Work out the finished part from the listing and answer in its coordinate system (mm). A direction names the side the tool comes from. Coordinates: 2 decimals unless noted, no trailing zeros. Order: outer loops, then holes, each group sorted by start corner. A loop starts at its lowest first (then second) coordinate and runs counter-clockwise, first axis right, second up. Notation, with made-up numbers: M -15,-16.5 L 38,-16.5 A28 cw 38,21.5 Z; hole C 60,86 d9. An arc over 180 degrees is marked long. Use a Markdown table: item, result.
from build123d import *

# Parameters (mm, degrees)
F0_W      = 127
F0_H      = 127
F1_DEPTH  = 63.5
F1_FACE_W = 127
F1_FACE_H = 127
F2_DEPTH  = 63.5
F3_W      = 76.2
F3_H      = 76.2
F4_DEPTH  = 8.89
F5_R      = 38.1
F6_DEPTH  = 8.89
F8_DEPTH  = 8.89
F10_DEPTH = 8.89
F12_DEPTH = 8.89
F13_R     = 5.08
F14_R     = 1.905
F15_DEPTH = 3.81


with BuildPart() as f1:
    # F0 (on Top) → F1 (new body)
    with BuildSketch(Plane.XY):
        Rectangle(F0_W, F0_H)
    extrude(amount=-F1_DEPTH)

    # F1_face (on face) → F2 (join)
    with BuildSketch(Plane.XY):
        Rectangle(F1_FACE_W, F1_FACE_H)
    extrude(amount=F2_DEPTH)

    # F3 (on face) → F4 (cut)
    with BuildSketch(Plane.XZ.offset(63.5)):
        Rectangle(F3_W, F3_H)
    extrude(amount=-F4_DEPTH, mode=Mode.SUBTRACT)

    # F5 (on face) → F6 (cut)
    with BuildSketch(Plane.YZ.offset(63.5)):
        Circle(F5_R)
    extrude(amount=-F6_DEPTH, mode=Mode.SUBTRACT)

    # F7 (on face) → F8 (cut)
    with BuildSketch(Plane(origin=(0, 63.5, 0), x_dir=(-1, 0, 0), z_dir=(0, 1, 0))):
        Polygon((-43.994091, -25.4), (43.994091, -25.4), (0, 50.8), align=None)
    extrude(amount=-F8_DEPTH, mode=Mode.SUBTRACT)

    # F9 (on face) → F10 (cut)
    with BuildSketch(Plane(origin=(-63.5, 0, 0), x_dir=(0, -1, 0), z_dir=(-1, 0, 0))):
        Polygon((21.997045, 38.1), (-21.997045, 38.1), (-43.994091, 0), (-21.997045, -38.1), (21.997045, -38.1), (43.994091, 0), align=None)
    extrude(amount=-F10_DEPTH, mode=Mode.SUBTRACT)

    # F11 (on face) → F12 (cut)
    with BuildSketch(Plane.XY.offset(63.5)):
        Polygon((0, 55.138838), (-12.37944, 17.038838), (-52.440151, 17.038838), (-20.030355, -6.508257), (-32.409796, -44.608257), (0, -21.061162), (32.409796, -44.608257), (20.030355, -6.508257), (52.440151, 17.038838), (12.37944, 17.038838), align=None)
    extrude(amount=-F12_DEPTH, mode=Mode.SUBTRACT)

    # F13
    f13_edges = [f1.edges().sort_by_distance(p)[0] for p in [
        (-63.5, 0, 63.5),
        (0, 63.5, 63.5),
        (63.5, 0, 63.5),
        (0, -63.5, 63.5),
        (63.5, -63.5, 0),
        (63.5, 63.5, 0),
        (63.5, 0, -63.5),
        (0, -63.5, -63.5),
        (-63.5, -63.5, 0),
        (0, 63.5, -63.5),
        (-63.5, 63.5, 0),
        (-63.5, 0, -63.5),
    ]]
    fillet(f13_edges, radius=F13_R)

    # F14 (on face) → F15 (cut)
    with BuildSketch(Plane(origin=(0, 0, 38.1), x_dir=(1, 0, 0), z_dir=(0, 0, -1))):
        with Locations((0, 58.912385)):
            Circle(F14_R)
    extrude(amount=-F15_DEPTH, mode=Mode.SUBTRACT)


solid = f1.part
1. Find the intervals of material crossed by probe 1 along Y at (x, z) = (0, 39.25); probe 2 along Z at (x, y) = (59, 0); probe 3 along Y at (x, z) = (29, 4.5), in increasing order.
Answers below:
| item | result |
|---|---|
| probe 1 | -63.5 to -60.82, -57.01 to 54.61 |
| probe 2 | -63.47 to -38.1, 38.1 to 63.47 |
| probe 3 | -54.61 to 63.5 |
2. Section B-B on y = 0 is taken. Determine the outline of the cut face in (x, z).
Answers below:
| item | result |
|---|---|
| outline | M -63.5,-58.42 A5.08 ccw -58.42,-63.5 L 58.42,-63.5 A5.08 ccw 63.5,-58.42 L 63.5,-38.1 L 54.61,-38.1 L 54.61,38.1 L 63.5,38.1 L 63.5,58.42 A5.08 ccw 58.42,63.5 L 28.99,63.5 L 28.99,54.61 L -28.99,54.61 L -28.99,63.5 L -58.42,63.5 A5.08 ccw -63.5,58.42 L -63.5,38.1 L -54.61,38.1 L -54.61,-38.1 L -63.5,-38.1 Z |
3. Section A-A on z = 2 is taken. Determine the outline of the cut face in (x, y).
Answers below:
| item | result |
|---|---|
| outline | M -63.5,-58.42 A5.08 ccw -58.42,-63.5 L -38.1,-63.5 L -38.1,-54.61 L 38.1,-54.61 L 38.1,-63.5 L 58.42,-63.5 A5.08 ccw 63.5,-58.42 L 63.5,-38.05 L 54.61,-38.05 L 54.61,38.05 L 63.5,38.05 L 63.5,58.42 A5.08 ccw 58.42,63.5 L 28.17,63.5 L 28.17,54.61 L -28.17,54.61 L -28.17,63.5 L -58.42,63.5 A5.08 ccw -63.5,58.42 L -63.5,42.84 L -54.61,42.84 L -54.61,-42.84 L -63.5,-42.84 Z |
4. Flat-ended cylindrical pins translate along their axes: P1, Ø4.5, axis at x = 27.5, z = 61, coming from the -Y side; P2, Ø10, axis at y = -6.5, z = -28, coming from the -X side; P3, Ø2, axis at x = 29.5, z = -9, coming from the -Y side. Find the tip coordinate at first contact, or state that the pin passes through.
Answers below:
| item | result |
|---|---|
| P1 | y = -63.49 |
| P2 | x = -54.61 |
| P3 | y = -54.61 |
5. Section C-C on x = 29 is taken. Determine the outline of the cut face in (y, z), then the cut area to 3 significant figures.
Answers below:
| item | result |
|---|---|
| outline | M -63.5,-58.42 A5.08 ccw -58.42,-63.5 L 58.42,-63.5 A5.08 ccw 63.5,-58.42 L 63.5,-25.4 L 54.61,-25.4 L 54.61,0.57 L 63.5,0.57 L 63.5,58.42 A5.08 ccw 58.42,63.5 L 17.04,63.5 L 17.04,54.61 L 0.01,54.61 L 0.01,63.5 L -34.11,63.5 L -34.11,54.61 L -42.13,54.61 L -42.13,63.5 L -58.42,63.5 A5.08 ccw -63.5,58.42 L -63.5,38.1 L -54.61,38.1 L -54.61,-38.1 L -63.5,-38.1 Z |
| area | 15,000 mm² |
6. Section D-D on z = -32 is taken. Determine the outline of the cut face in (x, y).
Answers below:
| item | result |
|---|---|
| outline | M -63.5,-58.42 A5.08 ccw -58.42,-63.5 L -38.1,-63.5 L -38.1,-54.61 L 38.1,-54.61 L 38.1,-63.5 L 58.42,-63.5 A5.08 ccw 63.5,-58.42 L 63.5,-20.68 L 54.61,-20.68 L 54.61,20.68 L 63.5,20.68 L 63.5,58.42 A5.08 ccw 58.42,63.5 L -58.42,63.5 A5.08 ccw -63.5,58.42 L -63.5,25.52 L -54.61,25.52 L -54.61,-25.52 L -63.5,-25.52 Z |
7. For a pull along Y with two mould halves and no side action, classify faces 6 (the face through (6.276, 35.822, 59.117)), 7 (the face through (-32, 17.039, 59)), 8 (the face through (-1, 63.5, -27)), 9 (the face through (21.69, 59.12, 13.23)) as +Y half, -Y half, draft (parallel to the pull), parting line (faces both ways), or undercut.
Answers below:
| item | result |
|---|---|
| face 6 | undercut |
| face 7 | undercut |
| face 8 | +Y half |
| face 9 | draft |
8. For faces 1 (the face through (0.818, -62.051, -61.972)), 2 (the face through (26.3, -25.8, 59.1)), 3 (the face through (-62.051, 0.818, -61.972)), 4 (the face through (-38.1, -59, -1)), 5 (the face through (-59.12, 33.15, -18.78)), determine the directions among +Z, -Z, +X, -X, +Y, -Y from which every point of the face is accessible in a straight line to the end or side of a thin tool.
Answers below:
| item | result |
|---|---|
| face 1 | -Z, +X, -X, -Y |
| face 2 | +Z |
| face 3 | -Z, -X, +Y, -Y |
| face 4 | -Y |
| face 5 | -X |
